Could you check a few things on this drawing? It's one solid part, dimensions in mm from its lowest x, y, z. Give positions to 0.01 mm unless a question says otherwise; leave off trailing zeros. Loops run counter-clockwise (first coordinate to the right, second up) from the corner with the lowest first, then second, coordinate; pieces in that order, holes last. Notation, with made-up numbers: (58.25, 87) - (109.25, 87) arc R22 cw to (109.25, 112) - close; hole circle Ø8 at (22, 89.25). An arc over 180 degrees is marked (long way). Use a Markdown table: item, result.
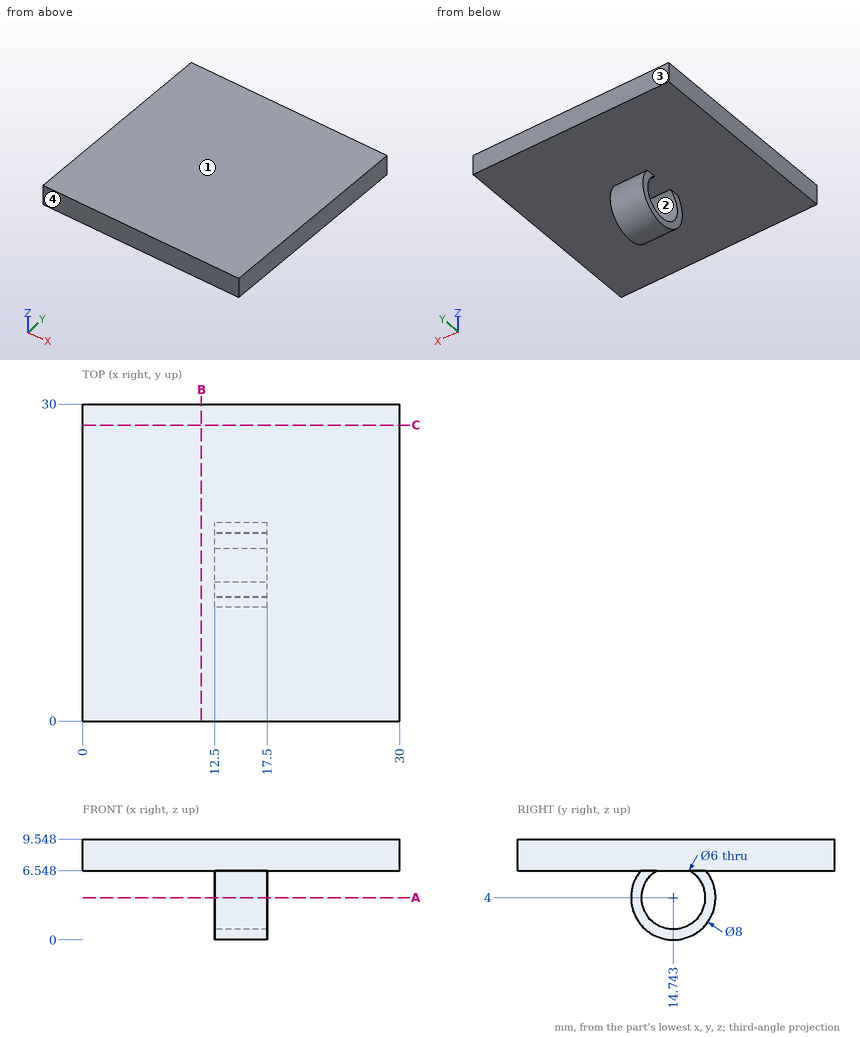
(1) Suppose I cut it at A-A on z = 4. Write out the boundary of the cut face in (x, y).
A:
| item | result |
|---|---|
| outline | (12.5, 10.74) - (17.5, 10.74) - (17.5, 11.74) - (12.5, 11.74) - close; (12.5, 17.74) - (17.5, 17.74) - (17.5, 18.74) - (12.5, 18.74) - close |
(2) We'd pull the mould along Y, two halves only. Please class the marked faces 1, 2, 3 and 4: pulls with the +Y half, pulls with the -Y half, needs draft (parallel to the pull), parting line crosses it, or undercut.
A:
| item | result |
|---|---|
| face 1 | needs draft |
| face 2 | undercut |
| face 3 | pulls with the +Y half |
| face 4 | pulls with the -Y half |
(3) Will these pins go through, and if not, where does the flat tip stop? pin 1 (2 mm diameter, centred on x = 17, z = 4, fed in from +Y); pin 2 (5 mm diameter, centred on x = 5.5, y = 16.5, fed in from -Z); pin 3 (2 mm diameter, centred on x = 17, z = 1, fed in from +Y).
A:
| item | result |
|---|---|
| pin 1 | y = 18.74 |
| pin 2 | z = 6.55 |
| pin 3 | y = 18.21 |
(4) If I drill on line 1 (Y direction, x = 14.7, z = 4); line 2 (Z direction, x = 25.5, y = 21.75); line 3 (Z direction, x = 14.5, y = 15.5), over which ranges is the centre line in solid material (lowest first)?
A:
| item | result |
|---|---|
| line 1 | 10.74 to 11.74, 17.74 to 18.74 |
| line 2 | 6.55 to 9.55 |
| line 3 | 0.07 to 1.1, 6.55 to 9.55 |
(5) Suppose I cut it at B-B on x = 11.25. Write out the boundary of the cut face in (y, z).
A:
| item | result |
|---|---|
| outline | (0, 6.55) - (30, 6.55) - (30, 9.55) - (0, 9.55) - close |
